Source: three-view drawing plus pictorial views. Frame: mm from the lowest corner of the part. A direction names the side the tool comes from. Give positions to 0.01 mm unless a question says otherwise; leave off trailing zeros. Order: outer loops, then holes, each group sorted by start corner. A loop starts at its lowest first (then second) coordinate and runs counter-clockwise, first axis right, second up. Notation, with made-up numbers: (83.25, -3.5) - (136.25, -3.5) arc R26 ccw to (136.25, 33.5) - close; hole circle Ø10 at (81, -7.5). An arc over 180 degrees is marked (long way). Answer in a Markdown table with one row per item. Add a question column.
1. Access query for the marked faces 1 and 2. Directions: +Z, -Z, +X, -X, +Y, -Y. A direction counts if a zero-diameter tool reaches every point of the face in a straight line with its end or side. Return the directions, or none.
2. Ray query, line 1 (X direction, y = 360, z = 232.5); line 2 (Z direction, x = 233.5, y = 569.5); line 3 (Y direction, x = 135, z = 1030.5). Return the intervals inside material, ascending. Write a range as [from, to].
3. Contact query for flat-ended pins moving along their axis: pin 1 (5 mm diameter, centred on y = 402, z = 834, fed in from -X); pin 2 (1 mm diameter, centred on x = 198, z = 682.5, fed in from -Y). Output: stop coordinate, or through.
4. Section query B-B on x = 112.5. Return loops of the section in (y, z), and give its area (3 significant figures).
5. Section query C-C on y = 68. Return loops of the section in (x, z).
6. Mould query, pull axis X, two halves, no side actions, for the marked faces 3, 4, 5 and 6. Classes: released by +X, released by -X, zero draft, split by the parting line, or undercut.
7. Section query A-A on z = 265. Return loops of the section in (x, y), and give its area (3 significant figures).
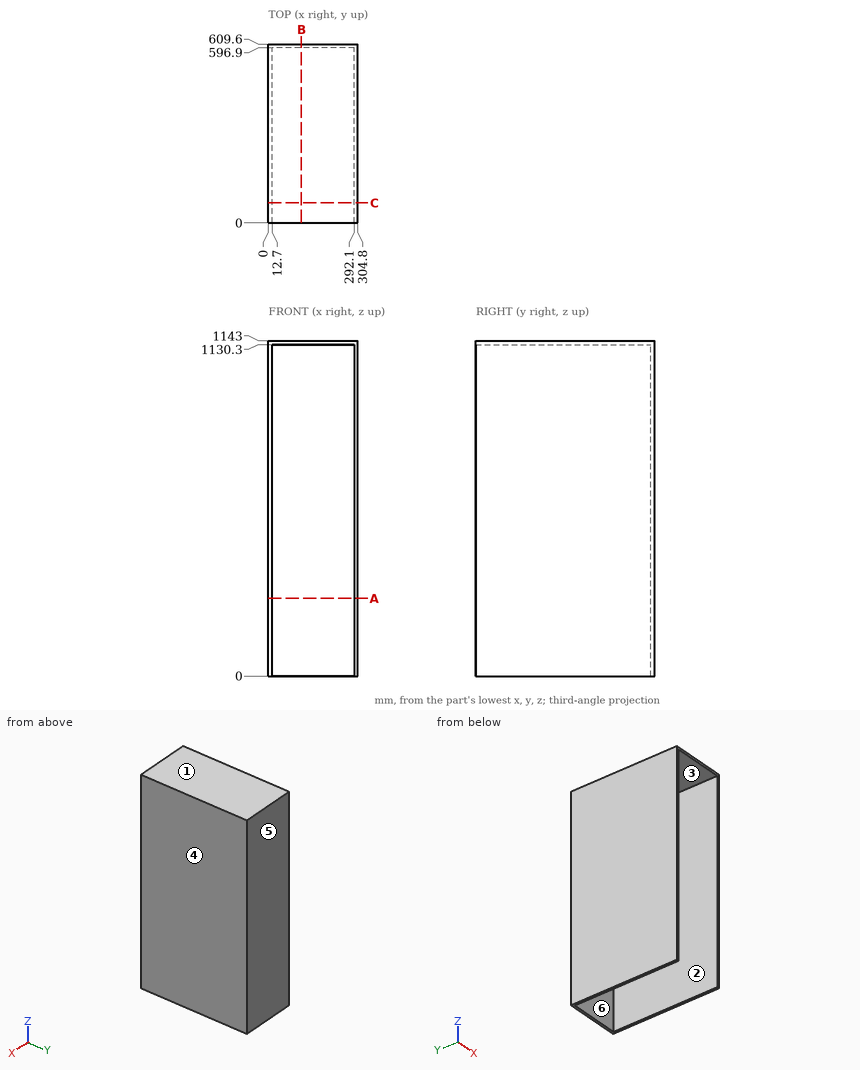
Answer:
| question | item | result |
|---|---|---|
| 1 | face 1 | +Z, +X, -X, +Y, -Y |
| 1 | face 2 | -Z, -Y |
| 2 | line 1 | x = [0, 12.7], [292.1, 304.8] |
| 2 | line 2 | z = [1130.3, 1143] |
| 2 | line 3 | y = [596.9, 609.6] |
| 3 | pin 1 | stops at x = 0 |
| 3 | pin 2 | stops at y = 596.9 |
| 4 | outline | (0, 1130.3) - (596.9, 1130.3) - (596.9, 0) - (609.6, 0) - (609.6, 1143) - (0, 1143) - close |
| 4 | area | 22,100 mm² |
| 5 | outline | (0, 0) - (12.7, 0) - (12.7, 1130.3) - (292.1, 1130.3) - (292.1, 0) - (304.8, 0) - (304.8, 1143) - (0, 1143) - close |
| 6 | face 3 | undercut |
| 6 | face 4 | released by +X |
| 6 | face 5 | zero draft |
| 6 | face 6 | undercut |
| 7 | outline | (0, 0) - (12.7, 0) - (12.7, 596.9) - (292.1, 596.9) - (292.1, 0) - (304.8, 0) - (304.8, 609.6) - (0, 609.6) - close |
| 7 | area | 19,000 mm² |
